Autodesk Inventor part; units mm, degrees
ref_plane "Work Plane2" through (-9.7807, 13.4392, 0.05) normal (-0.7071, -0.7071, 0) x (0, 0, 1)
ref_plane "YZ Plane" through (0, 0, 0) normal (1, 0, 0) x (0, 1, 0)
ref_plane "XZ Plane" through (0, 0, 0) normal (0, 1, 0) x (-1, 0, 0)
ref_plane "Work Plane1" through (-9.4272, 11.5884, 0.05) normal (0, 0, 1) x (1, 0, 0)
sketch "Sketch1" plane through (-9.4272, 11.5884, 0.05) normal (0, 0, 1) x (1, 0, 0)
  line L0 (-5.9698, 7.5884) -> (-5.9698, -7.5884)
  line L1 (-5.9698, -7.5884) -> (5.9698, -7.5884)
  line L2 (5.9698, -7.5884) -> (5.9698, 7.5884)
  line L3 (5.9698, 7.5884) -> (-5.9698, 7.5884)
  line L4 (-6.0698, 7.6884) -> (-6.0698, -7.6884)
  line L5 (-6.0698, -7.6884) -> (6.0698, -7.6884)
  line L6 (6.0698, -7.6884) -> (6.0698, 7.6884)
  line L7 (6.0698, 7.6884) -> (-6.0698, 7.6884)
  line L8 (-6.0698, -7.6884) -> (-21.0698, -7.6884)
  line L9 (-21.0698, -7.6884) -> (-21.0698, 9.3116)
  line L10 (6.0698, -7.6884) -> (11.0698, -7.6884)
  line L11 (11.0698, -7.6884) -> (11.0698, 9.3116)
  line L12 (11.0698, 9.3116) -> (-21.0698, 9.3116)
  point P0 (9.4272, -11.5884)
  dimension "d0" = 0.1
  dimension "d1" = 15
  dimension "d2" = 17
  dimension "d3" = 5
  dimension "d4" = 90
extrude "Extrusion1" add sketch "Sketch1" along normal blind 0.5 contours L3 L2 L1 L0 | L7 L6 L5 L4 | L4 L8 L9 L12 L11 L10 L6 L7
sketch "Sketch3" plane through (-9.4272, 11.5884, 0.55) normal (0, 0, 1) x (1, 0, 0)
  line L0 (-2.9698, 4.4671) -> (-0.8485, 6.5884)
  line L1 (2.2627, -0.7655) -> (-2.9698, 4.4671)
  line L2 (2.8284, -0.1998) -> (2.2627, -0.7655)
  line L3 (2.8284, 2.9115) -> (2.8284, -0.1998)
  line L4 (-0.8485, 6.5884) -> (2.8284, 2.9115)
  line L5 (5.6875, 2.1737) -> (6.0698, 1.7914)
  line L6 (6.0698, 1.7914) -> (6.0698, -4.8892)
  line L7 (6.0698, 7.6884) -> (6.0698, -7.5884)
  line L8 (6.0698, -4.8892) -> (5.1675, -5.7915)
  line L9 (5.1675, -5.7915) -> (-5.0912, 4.4671)
  line L10 (3.0284, 2.9943) -> (3.0284, -0.2826)
  line L11 (3.0284, -0.2826) -> (2.2627, -1.0483)
  line L12 (2.2627, -1.0483) -> (-3.2527, 4.4671)
  line L13 (-3.2527, 4.4671) -> (-0.8485, 6.8713)
  line L14 (-0.8485, 6.8713) -> (3.0284, 2.9943)
  line L15 (6.0698, -4.8892) -> (7.0698, -4.8892)
  line L16 (7.0698, -4.8892) -> (7.0698, -4.3892)
  line L17 (7.0698, -4.3892) -> (6.0698, -4.3892)
  line L18 (6.0698, -4.3892) -> (6.0698, -4.8892)
  line L19 (-11.0698, 9.4116) -> (11.0698, 9.4116)
  line L20 (-21.0698, -7.6884) -> (11.0698, -7.6884)
  line L21 (11.0698, 9.4116) -> (7.0698, 9.4116)
  line L22 (7.0698, 9.4116) -> (7.0698, -7.6884)
  line L23 (7.0698, -7.6884) -> (11.0698, -7.6884)
  line L24 (11.0698, -7.6884) -> (11.0698, 9.4116)
  line L25 (-5.0912, 4.4671) -> (-6.3481, 5.724)
  line L26 (-6.3481, 8.7553) -> (-0.8485, 8.7553)
  line L27 (-0.8485, 8.7553) -> (5.6875, 8.7553)
  line L28 (5.6875, 8.7553) -> (5.6875, 2.1737)
  line L29 (-5.0912, 4.4671) -> (-4.0305, 5.5278)
  line L30 (-1.9092, 7.6491) -> (-1.7678, 7.7905)
  line L31 (-6.3481, 5.724) -> (-6.3481, 5.724)
  line L32 (-6.3481, 5.724) -> (-6.3481, 8.7553)
  point P0 (9.4272, -11.5884)
  point P1 (11.0698, -7.6884)
  dimension "d10" = 1.5
  dimension "d11" = 1.5
  dimension "d14" = 0.2
  dimension "d15" = 1
  dimension "d16" = 0.5
extrude "Extrusion3" add sketch "Sketch3" along normal blind 9 contours L5 L6 L8 L9 L25 L32 L26 L27 L28 | L17 L16 L15 L6 | L22 L19 L24 L20 L16
sketch "Sketch4" plane through (-30.497, 3.9, 0.55) normal (0, -1, 0) x (1, 0, 0)
  line L0 (26.2373, 0) -> (14.7218, 0)
  line L1 (26.2373, 0) -> (26.2373, 9)
  line L2 (14.7218, 9) -> (26.2373, 9)
  line L3 (28.1397, 0) -> (0, 0)
  line L4 (0, 0) -> (28.1397, 0)
  line L5 (28.1397, 0) -> (28.1397, 0.3)
  line L6 (28.1397, 0.3) -> (0, 0.3)
  line L7 (0, 0.3) -> (0, 0)
  line L8 (14.7218, 0) -> (14.7218, 9)
  point P0 (30.497, -0.55)
  point P1 (1.736, 0)
  point P2 (18.1397, 0)
  dimension "d41" = 0.3
extrude "Extrusion4" cut sketch "Sketch4" against normal through all contours L0 L8 L6 L1 | L1 L6 L5 L3 | L3 L7 L6 L8
ref_plane "Work Plane3" through (1.6427, 4, -2.95) normal (1, 0, 0) x (0, 0, -1)
sketch "Sketch5" plane through (1.6427, 4, -2.95) normal (1, 0, 0) x (0, 0, -1)
  line L0 (-3, 16.9) -> (-3.5, 16.9)
  line L1 (-12.5, -0.1) -> (-12.5, 17)
  line L2 (-3, -0.1) -> (-12.5, -0.1)
  circle A0 centre (-8.4703, 13.9285) radius 1.4
  line L3 (-3, 16.9) -> (-3, -0.1)
  line L4 (-3.5, 17) -> (-3.5, 16.9)
  line L5 (-3.5, 17) -> (-12.5, 17)
  point P0 (-2.95, -4)
  dimension "d21" = 2.8
extrude "Extrusion5" cut sketch "Sketch5" against normal up to surface (5.3823 mm away) contours A0
sketch "Sketch6" plane through (-15.7753, 20.3438, 9.55) normal (0, 1, 0) x (1, 0, 0)
  circle A0 centre (8.0214, 3.9282) radius 3.2
  line L0 (8.0214, 3.9282) -> (8.0214, 4.8641) construction
  line L1 (11.2214, 3.9282) -> (11.2214, 4.8641)
  line L2 (4.8214, 4.8641) -> (4.8214, 3.9282)
  arc A1 (4.8214, 3.9282) -> (11.2214, 3.9282) centre (8.0214, 3.9282) ccw
  arc A2 (11.2214, 4.8641) -> (4.8214, 4.8641) centre (8.0214, 4.8641) ccw
  point P0 (15.7753, 9.55)
  point P1 (8.0214, 4.3961)
extrude "Extrusion6" cut sketch "Sketch6" against normal through all
sketch "Sketch7" plane through (-30.497, 3.9, 0.55) normal (-1, 0, 0) x (0, 0, 1)
  circle A0 centre (4.4299, 8.2054) radius 3.6733
  point P0 (-0.55, -3.9)
  point P1 (5.45, 8.2054)
ref_plane "Work Plane2" through (-9.7807, 13.4392, 0.05) normal (-0.7071, -0.7071, 0) x (0, 0, 1)
sketch "Sketch8" plane through (-4.2597, 5.7969, 9.55) normal (-0.7071, -0.7071, 0) x (-0.7071, 0.7071, 0)
  line L0 (16.2855, 8.7) -> (0, 8.7)
  line L1 (0, 8.7) -> (0, 0)
  line L2 (16.2855, 0) -> (0, 0)
  ellipse E0 centre (4.9415, 3.9282) end of major axis (9.4669, 3.9282) minor radius 3.2 (0.416, 3.9282) -> (9.4669, 3.9282) ccw
  ellipse E1 centre (4.9415, 4.8641) end of major axis (0.416, 4.8641) minor radius 3.2 (9.4669, 4.8641) -> (0.416, 4.8641) ccw
  line L3 (4.9374, 0.7098) -> (9.8018, 0.7098)
  line L4 (12.8018, 3.7098) -> (12.8018, 5.1494)
  line L5 (9.8018, 8.1494) -> (4.9374, 8.1494)
  line L6 (1.9374, 5.1494) -> (1.9374, 3.7098)
  arc A0 (9.8018, 0.7098) -> (12.8018, 3.7098) centre (9.8018, 3.7098) ccw
  arc A1 (12.8018, 5.1494) -> (9.8018, 8.1494) centre (9.8018, 5.1494) ccw
  arc A2 (4.9374, 8.1494) -> (1.9374, 5.1494) centre (4.9374, 5.1494) ccw
  arc A3 (1.9374, 3.7098) -> (4.9374, 0.7098) centre (4.9374, 3.7098) ccw
  line L7 (9.4669, 4.8641) -> (9.4669, 3.9282)
  line L8 (16.2855, 8.7) -> (16.2855, 0)
  line L9 (0.416, 3.9282) -> (0.416, 4.8641)
  point P0 (-7.1111, 9.55)
  dimension "d42" = 3
extrude "Extrusion8" cut sketch "Sketch8" against normal up to surface (1.3 mm away) contours A3 L6 A2 E1 L7 E0 | E0 L7 E1 A2 L5 A1 L4 A0 L3 A3
ref_plane "Work Plane4" through (-9.4272, 11.5884, -2.95) normal (0, 0, -1) x (-1, 0, 0)
ref_plane "Work Plane7" through (-6.3987, 11.3058, 7.8996) normal (0, 1, 0) x (1, 0, 0)
ref_plane "Work Plane5" through (-3.3573, 3.9, 0.05) normal (0, -1, 0) x (1, 0, 0)
sketch "Sketch16" plane through (-3.3573, 3.9, 0.05) normal (0, -1, 0) x (1, 0, 0)
  line L0 (1, 0.5) -> (1, 9.5)
  line L1 (-27.1397, 0.5) -> (1, 0.5)
  line L2 (5, 0) -> (-27.1397, 0)
  line L3 (5, 0) -> (5, 9.5)
  line L4 (1, 9.5) -> (5, 9.5)
  line L5 (5, 0) -> (-27.1397, 0)
  line L6 (-12.1397, 0.5) -> (0, 0.5)
  line L7 (5, 0) -> (-27.1397, 0)
  line L8 (-27.1397, 0.5) -> (1, 0.5)
  line L9 (-27.1397, 0) -> (-27.1397, 0.5)
  line L10 (-12.1397, 0) -> (-12.1397, 0.5)
  circle A0 centre (5.0158, 8.95) radius 1
  circle A1 centre (-16.4842, -6.55) radius 1
  circle A2 centre (-22.9842, 13.95) radius 1
  line L11 (-27.1287, 16.95) -> (8.0158, 16.95)
  line L12 (8.0158, 16.95) -> (8.0158, 0)
  line L13 (8.0158, 0) -> (-27.1287, 0)
  line L14 (-27.1287, 0) -> (-27.1287, 16.95)
  circle A3 centre (-22.9842, 13.95) radius 1
  circle A4 centre (5.0158, 8.95) radius 1
  line L15 (0.9985, 0.5) -> (-17.4842, 0.5)
  line L16 (-17.4842, 0.5) -> (-17.4842, 10.2078)
  line L17 (-17.4842, 10.2078) -> (0.9985, 10.2078)
  line L18 (0.9985, 10.2078) -> (0.9985, 0.5)
  line L19 (-27.1397, 0) -> (-27.1397, 0.5)
  point P0 (3.3573, -0.05)
  point P1 (0, 0)
  dimension "d53" = 3
  dimension "d54" = 3
  dimension "d55" = 2
  dimension "d56" = 2
extrude "Extrusion15" add sketch "Sketch16" against normal blind 4 contours L0 L4 A0 L3 L2 L10 L1 | L18 L17 L16 L1 L14 L11 L12 L13 L3 A0 L4 | L4 L3 A0 | L10 L2 L14 L1 | L14 L2 L9 L1 picked at (4.9217, 8.4773)
ref_plane "Work Plane6" through (-29.3415, 3.9, 17) normal (0, -1, 0) x (1, 0, 0)
sketch "Sketch17" plane through (-29.3415, 3.9, 17) normal (0, -1, 0) x (1, 0, 0)
  arc A0 (30.9842, -8.9999) -> (30.1648, -7.45) centre (31, -8) ccw
  circle A1 centre (31, -8) radius 1
  point P0 (29.3415, -17)
extrude "Extrusion16" cut sketch "Sketch17" against normal through all
sketch "Sketch18" plane through (1.6427, 20.9, 0.55) normal (1, 0, 0) x (0, 0, -1)
  line L0 (0.5, 0) -> (0.5, -13)
  line L1 (0.5, 0) -> (0, 0)
  line L2 (0, 0.1) -> (0, 0)
  line L3 (0, 0.1) -> (-7.4501, 0.1)
  line L4 (-9, -7.1378) -> (-9, -0.5562)
  line L5 (-0.3, -7.1378) -> (-9, -7.1378)
  circle A0 centre (-4.1776, -3.2963) radius 1.45
  line L6 (-0.3, -0.5562) -> (-9, -0.5562)
  line L7 (-7.4501, 0.1) -> (-7.4501, -13)
  line L8 (-7.4501, -13) -> (0.5, -13)
  line L9 (-0.3, -7.1378) -> (-0.3, -0.5562)
  point P0 (0.55, -20.9)
  dimension "d61" = 2.9
extrude "Extrusion17" cut sketch "Sketch18" against normal up to surface (5.3823 mm away) contours A0
sketch "Sketch19" plane through (-9.4272, 11.5884, 9.55) normal (0, 0, 1) x (1, 0, 0)
  line L0 (7.0684, -4.8892) -> (7.0684, -4.3892)
  line L1 (7.0684, -4.3892) -> (6.0698, -4.3892)
  line L2 (6.0698, -4.3892) -> (6.0698, 1.7914)
  line L3 (6.0698, 1.7914) -> (5.6875, 2.1737)
  line L4 (5.6875, 2.1737) -> (5.6875, 8.7553)
  line L5 (5.6875, 8.7553) -> (-6.3481, 8.7553)
  line L6 (-6.3481, 8.7553) -> (-6.3481, 5.724)
  line L7 (-6.3481, 5.724) -> (5.1675, -5.7915)
  line L8 (5.1675, -5.7915) -> (6.0698, -4.8892)
  line L9 (6.0698, -4.8892) -> (7.0684, -4.8892)
  line L10 (3.0284, -0.2826) -> (2.2627, -1.0483)
  line L11 (2.2627, -1.0483) -> (-3.2527, 4.4671)
  line L12 (-3.2527, 4.4671) -> (-0.8485, 6.8713)
  line L13 (-0.8485, 6.8713) -> (3.0284, 2.9943)
  line L14 (3.0284, 2.9943) -> (3.0284, -0.2826)
  line L15 (2.2627, -1.0483) -> (-3.2527, 4.4671)
  line L16 (2.1513, -0.9369) -> (2.1513, -2.7754)
  line L17 (-6.3481, 5.724) -> (5.1675, -5.7915)
  line L18 (5.6875, 2.1737) -> (5.6875, 8.7553)
  line L19 (2.1513, -2.7754) -> (6.0698, -2.7754)
  line L20 (2.8027, 3.22) -> (5.6875, 3.22)
  point P0 (9.4272, -11.5884)
extrude "Extrusion18" add sketch "Sketch19" against normal up to surface (8.7 mm away) contours L9 L8 L7 L19 L2 L1 L0 | L19 L16 L11 L10 L14 L13 L20 L4 L3 L2
sketch "Sketch20" plane through (-9.4272, 11.5884, 0.55) normal (0, 0, 1) x (1, 0, 0)
  line L0 (7.0684, -7.6884) -> (7.0684, -3.6884)
  line L1 (7.0684, -3.6884) -> (7.0698, -3.6884)
  line L2 (7.0698, -3.6884) -> (7.0698, 9.3116)
  line L3 (7.0698, 9.3116) -> (-21.0698, 9.3116)
  line L4 (-21.0698, 9.3116) -> (-21.0698, -7.6884)
  line L5 (-21.0698, -7.6884) -> (-21.0589, -7.6884)
  line L6 (-21.0589, -7.6884) -> (-21.0589, -3.6884)
  line L7 (-21.0589, -3.6884) -> (-11.4143, -3.6884)
  line L8 (-11.4143, -3.6884) -> (-11.4143, -7.6884)
  line L9 (-11.4143, -7.6884) -> (7.0684, -7.6884)
  line L10 (-21.0698, 9.3116) -> (-13.0698, 9.3116)
  line L11 (-13.0698, 9.3116) -> (-13.0698, 4.3116)
  line L12 (-13.0698, 4.3116) -> (-21.0698, 4.3116)
  line L13 (-21.0698, 4.3116) -> (-21.0698, 9.3116)
  point P0 (9.4272, -11.5884)
  dimension "d66" = 8
  dimension "d67" = 5
extrude "Extrusion19" add sketch "Sketch20" along normal up to surface (9 mm away) contours L11 L12 L4 L3
sketch "Sketch21" plane through (-30.497, 3.9, 0.05) normal (-1, 0, 0) x (0, 0, 1)
  line L0 (0, 17) -> (9.5, 17)
  line L1 (0, 0) -> (0, 17)
  line L2 (0, 0) -> (0.5, 0)
  line L3 (0.5, 12) -> (0.5, 0)
  line L4 (0.5, 12) -> (9.5, 12)
  line L5 (9.5, 12) -> (9.5, 17)
  circle A0 centre (5, 14.5) radius 0.95
  point P0 (-0.05, -3.9)
  dimension "d70" = 1.9
extrude "Extrusion20" cut sketch "Sketch21" against normal up to surface (8 mm away) contours A0
properties part number "cellSTORM_dichroic_mirror_adjuster_tmp"
Geometry check sheet. Reference: the model listing, model coordinates, mm. A direction names the side the tool comes from. Coordinates: 2 decimals unless noted, no trailing zeros. Loops run counter-clockwise (first coordinate to the right, second up) from the corner with the lowest first, then second, coordinate; pieces in that order, holes last.
Item 1: Sectioned sample at A-A, the plane x = -19. Record the boundary of the cut face in (y, z), then the cut area to 3 significant figures.
Item 2: Sectioned sample at D-D, the plane x = -8.5. Record the boundary of the cut face in (y, z).
Item 3: Sectioned sample at B-B, the plane z = 14. Record the boundary of the cut face in (x, y), then the cut area to 3 significant figures.
Item 4: Access from +Z, -Z, +X, -X, +Y, -Y to the whole of each face (thin tool, end or side, straight path). Record for faces 4 (the face through (-0.3, 18.5, 6.8)), 5 (the face through (-3.802, 6.254, 5.139)), 6 (the face through (-3, 7.199, 5)), 7 (the face through (-10.954, 19, 5)).
Item 5: Sectioned sample at C-C, the plane x = -27. Record the boundary of the cut face in (y, z), then the cut area to 3 significant figures.
Item 6: Go/stop test with flat-tipped pins: pin 1 Ø0.6 at (x, z) = (-5.5, 4.5) entering from +Y; pin 2 Ø8 at (x, y) = (-12.5, 14) entering from +Z; pin 3 Ø4 at (y, z) = (13.5, 6) entering from +X. Record where each tip stops, or that it passes through.
Item 7: Thickness scan on line 1 (Z direction, x = -12.5, y = 20); line 2 (Y direction, x = -23, z = 5.25); line 3 (X direction, y = 12.25, z = 4.75). Record the ranges inside material, lowest first.
Item 8: Release check for a two-part mould opening along Z. For faces 1 (the face through (-4.554, 18, 5)), 2 (the face through (-1, 15, 9.55)), 3 (the face through (-25, 20.9, 4)) record: released by +Z, released by -Z, zero draft, split by the parting line, or undercut.
Check result:
1. outline: (3.9, 0.05) - (20.9, 0.05) - (20.9, 0.55) - (3.9, 0.55) - close; (3.9, 10.26) - (7.9, 10.26) - (7.9, 17) - (3.9, 17) - close
1. area: 35.5 mm2
2. outline: (3.9, 0.05) - (20.9, 0.05) - (20.9, 0.55) - (3.9, 0.55) - close; (3.9, 10.26) - (7.9, 10.26) - (7.9, 17) - (3.9, 17) - close; (10.04, 0.85) - (11.88, 0.85) - (11.88, 1.4) - (10.04, 1.4) - close; (10.04, 8.84) - (11.88, 8.84) - (11.88, 9.55) - (10.04, 9.55) - close; (16.68, 0.85) - (20.34, 0.85) - (20.34, 1.57) - (16.68, 1.57) - close; (16.68, 8.73) - (20.34, 8.73) - (20.34, 9.55) - (16.68, 9.55) - close
3. outline: (-30.49, 3.9) - (-27.34, 3.9) - (-27.34, 7.9) - (-30.49, 7.9) - close; (-25.34, 3.9) - (4.66, 3.9) - (4.66, 7.9) - (-25.34, 7.9) - close
3. area: 133 mm2
4. face 4: +X
4. face 5: -Y
4. face 6: +Y
4. face 7: +Y, -Y
5. outline: (3.9, 0.05) - (20.9, 0.05) - (20.9, 9.55) - (15.9, 9.55) - (15.9, 0.55) - (7.9, 0.55) - (7.9, 13.25) - (3.9, 13.25) - close; (3.9, 14.75) - (7.9, 14.75) - (7.9, 17) - (3.9, 17) - close; hole circle Ø1.9 at (18.4, 5.05)
5. area: 110 mm2
6. pin 1: stops at y = 14.81
6. pin 2: stops at z = 9.55
6. pin 3: stops at x = 1.64
7. line 1: z = 0.05 to 0.55, 0.85 to 9.55
7. line 2: y = 3.9 to 7.9, 15.9 to 17.47, 19.33 to 20.9
7. line 3: x = -6.4 to -3.36, -2.36 to 1.64
8. face 1: undercut
8. face 2: released by +Z
8. face 3: zero draft
